For this review, take the finished solid that the model builds, in its own axes (mm). A direction names the side the tool comes from. Give positions to 0.01 mm unless a question says otherwise; leave off trailing zeros. Loops run counter-clockwise (first coordinate to the right, second up) from the corner with the lowest first, then second, coordinate; pieces in that order, holes last. Notation, with made-up numbers: (-37, 21.5) - (-4, 21.5) arc R11 cw to (-4, 28.5) - close; hole circle Ø5 at (9, -30). An arc over 180 degrees is marked (long way). Answer in a Markdown table with one row per item.
Autodesk Inventor part; units mm, degrees
ref_plane "YZ Plane" through (0, 0, 0) normal (1, 0, 0) x (0, 1, 0)
ref_plane "XZ Plane" through (0, 0, 0) normal (0, 1, 0) x (-1, 0, 0)
ref_plane "XY Plane" through (0, 0, 0) normal (0, 0, 1) x (1, 0, 0)
sketch "Sketch1" plane through (0, 0, 0) normal (0, 0, 1) x (1, 0, 0)
  line L0 (0, 0) -> (25.4, 0)
  line L1 (25.4, 0) -> (25.4, 25.4)
  line L2 (25.4, 25.4) -> (0, 25.4)
  line L3 (0, 25.4) -> (0, 0)
  dimension "d0" = 25.4
  dimension "d1" = 25.4
extrude "Extrusion1" add sketch "Sketch1" along normal blind 635
shell "Shell1" thickness 3.175 removed faces 2 at (8.4667, 16.9333, 0) at (16.9333, 8.4667, 635)
sketch "Sketch2" plane through (0, 25.4, 0) normal (0, 1, 0) x (1, 0, 0)
  line L0 (0, -635) -> (25.4, -635)
  line L1 (25.4, 0) -> (0, 0)
  line L2 (0, 0) -> (0, -635)
  circle A0 centre (12.7, -50.8) radius 3.175
  circle A1 centre (12.7, -101.6) radius 3.175
  circle A2 centre (12.7, -533.4) radius 3.175
  circle A3 centre (12.7, -584.2) radius 3.175
  dimension "d7" = 50.8
  dimension "d8" = 50.8
  dimension "d9" = 12.7
  dimension "d10" = 12.7
  dimension "d11" = 6.35
  dimension "d12" = 6.35
  dimension "d13" = 12.7
  dimension "d14" = 12.7
  dimension "d15" = 50.8
  dimension "d16" = 50.8
  dimension "d17" = 6.35
  dimension "d18" = 6.35
extrude "Extrusion2" cut sketch "Sketch2" against normal through all
sketch "Sketch3" plane through (0, 25.4, 0) normal (0, 1, 0) x (1, 0, 0)
  line L0 (25.4, 0) -> (0, 0)
  line L1 (0, 0) -> (0, -635)
  line L2 (12.7, 0) -> (12.7, -254) construction
  line L3 (12.7, -254) -> (12.7, -381) construction
  circle A0 centre (12.7, -254) radius 2.3813
  circle A1 centre (12.7, -381) radius 2.3813
  dimension "d21" = 4.7625
  dimension "d22" = 4.7625
  dimension "d23" = 127
  dimension "d24" = 254
extrude "Extrusion3" cut sketch "Sketch3" against normal through all
properties part number "DriveTrain_SideRail" material "Aluminum-6061"
1. We need section A-A, the plane z = 486.5. Give the boundary of the cut face in (x, y) (3 decimals).
Values:
| item | result |
|---|---|
| outline | (0, 0) - (25.4, 0) - (25.4, 25.4) - (0, 25.4) - close; hole (3.175, 3.175) - (22.225, 3.175) - (22.225, 22.225) - (3.175, 22.225) - close |
2. Mouldability with a two-part tool opening along Y and no side actions: class faces 3 (the face through (25.4, 13, 313)), 4 (the face through (13, 0, 313)), 5 (the face through (3.175, 13, 313)), 6 (the face through (22.225, 13, 313)) as released by +Y, released by -Y, zero draft, split by the parting line, or undercut.
Values:
| item | result |
|---|---|
| face 3 | zero draft |
| face 4 | released by -Y |
| face 5 | undercut |
| face 6 | undercut |
3. We need section B-B, the plane y = 16.25. Give the boundary of the cut face in (x, z) (3 decimals), and give its area (3 significant figures).
Values:
| item | result |
|---|---|
| outline | (0, 0) - (3.175, 0) - (3.175, 635) - (0, 635) - close; (22.225, 0) - (25.4, 0) - (25.4, 635) - (22.225, 635) - close |
| area | 4,030 mm^2 |
4. Wall thickness on line 1 (X direction, y = 2.05, z = 533.4) (3 decimals); line 2 (X direction, y = 3.75, z = 252.5) (3 decimals): over which ranges is each line inside the solid? List them lowest first. Write a range as [from, to].
Values:
| item | result |
|---|---|
| line 1 | x = [0, 9.525], [15.875, 25.4] |
| line 2 | x = [0, 3.175], [22.225, 25.4] |
5. Clearance check with a flat-ended pin moving along its axis: pin 1 (4 mm diameter, centred on x = 12.7, z = 50.8, fed in from -Y). State where the tip first meets the part, or that it passes through.
Values:
| item | result |
|---|---|
| pin 1 | passes through |
6. For faces 1 (the face through (13, 22.225, 313)), 2 (the face through (0, 13, 313)), list the 3-axis set-ups (+Z, -Z, +X, -X, +Y, -Y) from which the entire face can be reached by the end or side of a thin tool; tool diameter is ignored.
Values:
| item | result |
|---|---|
| face 1 | +Z, -Z |
| face 2 | +Z, -Z, -X, +Y, -Y |
